Geometry: final body of the model. Coordinates: model frame, mm. A direction names the side the tool comes from. Round coordinates to 2 decimals unless told otherwise and drop trailing zeros. Loops run counter-clockwise (first coordinate to the right, second up) from the corner with the lowest first, then second, coordinate; pieces in that order, holes last. Notation, with made-up numbers: (68.5, 86) - (114.5, 86) arc R8 ccw to (114.5, 90) - close; hole circle Ø1 at (43, 3.25). An arc over 180 degrees is marked (long way). Return JSON: item names as keys, results as strings. Group by question number.
1. Section B-B on z = 73.5. Return loops of the section in (x, y), and give its area (3 significant figures).
2. Material intervals for probe 1 along Z at (x, y) = (-12, 13); probe 2 along Y at (x, z) = (0.5, -0.5); probe 3 along X at (y, z) = (-0.5, 26), sorted ascending.
3. Set-up query: faces 1 (the face through (0, 0, 84.5)), 2 (the face through (8, -4, 66.5)), 3 (the face through (-0.54, 2.44, -11.86)). Return all of +Z, -Z, +X, -X, +Y, -Y with unobstructed straight access to the full face (end or side cutting, diameter ignored); none if empty.
4. Section A-A on y = 0. Return loops of the section in (x, z).
5. First-contact query: pin 1 Ø1 at (y, z) = (-11, 37) entering from -X; pin 2 Ø5 at (x, y) = (-8, -12) entering from -Z; pin 3 Ø1.5 at (y, z) = (-13.5, 47.5) entering from +X. Flat tips, straight axial feed; report the tip coordinate or a pass-through.
6. Section C-C on z = 50.5. Return loops of the section in (x, y), and give its area (3 significant figures).
from build123d import *

# Parameters (mm, degrees)
SKETCH_R     = 22.5
PAD_DEPTH    = 66.5
FILLET_R     = 3
SKETCH001_R  = 8.75
PAD001_DEPTH = 2
FILLET001_R  = 1
SKETCH002_R  = 2.5
PAD002_DEPTH = 16
FILLET002_R  = 1
SKETCH003_R  = 8.75
PAD003_DEPTH = 2
FILLET003_R  = 1
SKETCH004_R  = 2.5
PAD004_DEPTH = 20


with BuildPart() as part:
    # Sketch → Pad (new body)
    with BuildSketch(Plane.XY):
        with Locations((-0.540205, 0)):
            Circle(SKETCH_R)
    extrude(amount=PAD_DEPTH)

    # Fillet
    fillet_edges = [part.edges().sort_by_distance(p)[0] for p in [
        (-23.040205, 0, 66.5),
    ]]
    fillet(fillet_edges, radius=FILLET_R)

    # Sketch001 (on Face4 of Fillet) → Pad001 (join)
    with BuildSketch(Plane.XY.offset(66.5)):
        Circle(SKETCH001_R)
    extrude(amount=PAD001_DEPTH)

    # Fillet001
    fillet001_edges = [part.edges().sort_by_distance(p)[0] for p in [
        (-8.75, 0, 68.5),
    ]]
    fillet(fillet001_edges, radius=FILLET001_R)

    # Sketch002 (on Face4 of Fillet001) → Pad002 (join)
    with BuildSketch(Plane.XY.offset(68.5)):
        Circle(SKETCH002_R)
    extrude(amount=PAD002_DEPTH)

    # Fillet002
    fillet002_edges = [part.edges().sort_by_distance(p)[0] for p in [
        (-2.5, 0, 84.5),
    ]]
    fillet(fillet002_edges, radius=FILLET002_R)

    # Sketch003 (on Face10 of Fillet002) → Pad003 (join)
    with BuildSketch(Plane(origin=(0, 0, 0), x_dir=(1, 0, 0), z_dir=(0, 0, -1))):
        Circle(SKETCH003_R)
    extrude(amount=PAD003_DEPTH)

    # Fillet003
    fillet003_edges = [part.edges().sort_by_distance(p)[0] for p in [
        (-8.75, 0, -2),
    ]]
    fillet(fillet003_edges, radius=FILLET003_R)

    # Sketch004 (on Face4 of Fillet003) → Pad004 (join)
    with BuildSketch(Plane(origin=(0, 0, -2), x_dir=(1, 0, 0), z_dir=(0, 0, -1))):
        Circle(SKETCH004_R)
    extrude(amount=PAD004_DEPTH)


solid = part.part
Taken from the geometry:
{
 "1": {"outline": "circle Ø5 at (0, 0)", "area": "19.6 mm2"},
 "2": {"probe 1": "0 to 66.5", "probe 2": "-8.74 to 8.74", "probe 3": "-23.03 to 21.95"},
 "3": {"face 1": "+Z, +X, -X, +Y, -Y", "face 2": "+Z", "face 3": "-Z"},
 "4": {"outline": "(-23.04, 0) - (-8.75, 0) - (-8.75, -1) arc R1 ccw to (-7.75, -2) - (-2.5, -2) - (-2.5, -22) - (2.5, -22) - (2.5, -2) - (7.75, -2) arc R1 ccw to (8.75, -1) - (8.75, 0) - (21.96, 0) - (21.96, 63.5) arc R3 ccw to (18.96, 66.5) - (8.75, 66.5) - (8.75, 67.5) arc R1 ccw to (7.75, 68.5) - (2.5, 68.5) - (2.5, 83.5) arc R1 ccw to (1.5, 84.5) - (-1.5, 84.5) arc R1 ccw to (-2.5, 83.5) - (-2.5, 68.5) - (-7.75, 68.5) arc R1 ccw to (-8.75, 67.5) - (-8.75, 66.5) - (-20.04, 66.5) arc R3 ccw to (-23.04, 63.5) - close"},
 "5": {"pin 1": "x = -20.44", "pin 2": "z = 0", "pin 3": "x = 18"},
 "6": {"outline": "circle Ø45 at (-0.54, 0)", "area": "1,590 mm2"}
}
